```python
from build123d import *
from build123d.topology import SkipClean

# Parameters (mm, degrees)
SKETCH_1_R          = 22
SKETCH_1_R_2        = 11.15
SKETCH_1_R_3        = 2.7
EXTRUDE_1_DEPTH     = 10
EXTRUDE_START       = -10
EXTRUDE_2_DEPTH     = 10
CUT_EXTRUDE_START   = -10
CUT_EXTRUDE_1_DEPTH = 10
SKETCH_4_W          = 20
SKETCH_4_H          = 20
EXTRUDE_3_DEPTH     = 15
CHAMFER_2_SIZE      = 10
CHAMFER_4_SIZE      = 1
SKETCH_6_R          = 1.7
CUT_EXTRUDE_3_DEPTH = 92.290744328
CHAMFER_6_SIZE      = 1


with BuildPart() as part:
    # ｽｹｯﾁ1 → ﾎﾞｽ - 押し出し1 (new body)
    with BuildSketch(Plane.XY):
        Circle(SKETCH_1_R)
        Circle(SKETCH_1_R_2, mode=Mode.SUBTRACT)
        with Locations((-8.75, -15.155444566)):
            Circle(SKETCH_1_R_3, mode=Mode.SUBTRACT)
        with Locations((17.5, 0)):
            Circle(SKETCH_1_R_3, mode=Mode.SUBTRACT)
        with Locations((-8.75, 15.155444566)):
            Circle(SKETCH_1_R_3, mode=Mode.SUBTRACT)
    extrude(amount=EXTRUDE_1_DEPTH)

    # ｽｹｯﾁ2 → ﾎﾞｽ - 押し出し2 (add)
    with BuildSketch(Plane.XY.offset(10).offset(EXTRUDE_START)):
        with BuildLine():
            ThreePointArc((0, -22), (-22, 0), (0, 22))
            Line((0, 22), (-85, 22))
            Line((-85, 22), (-85, -22))
            Line((-85, -22), (0, -22))
        make_face()
    extrude(amount=EXTRUDE_2_DEPTH)

    # ｽｹｯﾁ3 → ｶｯﾄ - 押し出し1 (cut)
    with BuildSketch(Plane.XY.offset(10).offset(CUT_EXTRUDE_START)):
        with BuildLine():
            Line((-85, 22), (-85, 10))
            Line((-85, 10), (-19.595917942, 10))
            ThreePointArc((-19.595917942, 10), (-11.489125293, 18.761663039), (0, 22))
            Line((0, 22), (-85, 22))
        make_face()
        with BuildLine():
            Line((-19.595917942, -10), (-85, -10))
            Line((-85, -10), (-85, -22))
            Line((-85, -22), (0, -22))
            ThreePointArc((0, -22), (-11.489125293, -18.761663039), (-19.595917942, -10))
        make_face()
    extrude(amount=CUT_EXTRUDE_1_DEPTH, mode=Mode.SUBTRACT)

    # ｽｹｯﾁ4 → ﾎﾞｽ - 押し出し3 (add)
    with BuildSketch(Plane(origin=(0, 0, 0), x_dir=(-1, 0, 0), z_dir=(0, 0, -1))):
        with Locations((75, 0)):
            Rectangle(SKETCH_4_W, SKETCH_4_H)
    extrude(amount=EXTRUDE_3_DEPTH)

    # 面取り2
    chamfer_2_edges = [part.edges().sort_by_distance(p)[0] for p in [
        (-65, 0, 0),
    ]]
    chamfer(chamfer_2_edges, length=CHAMFER_2_SIZE)

    # 面取り4
    chamfer_4_edges = [part.edges().sort_by_distance(p)[0] for p in [
        (22, 0, 10),
        (-52.297958971, 10, 10),
        (-52.297958971, -10, 10),
    ]]
    chamfer(chamfer_4_edges, length=CHAMFER_4_SIZE)

    # ｽｹｯﾁ6 → ｶｯﾄ - 押し出し3 (cut, through all)
    with SkipClean():  # the faces are left unmerged after this step: merging them gives an invalid solid
        with BuildSketch(Plane(origin=(0, 0, -15), x_dir=(-1, 0, 0), z_dir=(0, 0, -1))):
            with Locations((80, 5)):
                Circle(SKETCH_6_R)
            with Locations(Location((70, 5, 0), (0, 0, 180))):
                Circle(SKETCH_6_R)
            with Locations((70, -5)):
                Circle(SKETCH_6_R)
            with Locations(Location((80, -5, 0), (0, 0, 180))):
                Circle(SKETCH_6_R)
        extrude(amount=-CUT_EXTRUDE_3_DEPTH, mode=Mode.SUBTRACT)

    # 面取り6
    chamfer_6_edges = [part.edges().sort_by_distance(p)[0] for p in [
        (-85, 0, 10),
    ]]
    chamfer(chamfer_6_edges, length=CHAMFER_6_SIZE)


solid = part.part
```
Geometry: final body of the model. Coordinates: model frame, mm. A direction names the side the tool comes from. Coordinates: 2 decimals unless noted, no trailing zeros. Order: outer loops, then holes, each group sorted by start corner. A loop starts at its lowest first (then second) coordinate and runs counter-clockwise, first axis right, second up. Notation, with made-up numbers: (14, 50.5) -> (32, 50.5) arc R18 ccw to (32, 62.5) -> close; hole circle Ø6 at (-27, -33.75). An arc over 180 degrees is marked (long way). Write item = value, one per line.
(1) Pin query (flat end, axial travel): pin 1 Ø6 at (x, z) = (-38.5, 2) entering from -Y; pin 2 Ø8.5 at (x, y) = (17.5, 0) entering from +Z; pin 3 Ø22 at (x, y) = (-18.5, 4) entering from -Z; pin 4 Ø5.5 at (y, z) = (3.5, -12.5) entering from +X. Return the tip coordinate at first contact, or that it passes through.
Solved:
pin_1 = -10
pin_2 = 10
pin_3 = 0
pin_4 = -64.75
(2) Line query: line 1 (Y direction, x = -70, z = -8); line 2 (X direction, y = -4, z = -2); line 3 (X direction, y = 1.5, z = 8) (3 decimals). Output: solid intervals per line, ascending.
Solved:
line_1 = -10 to -6.7, -3.3 to 3.3, 6.7 to 10
line_2 = -85 to -81.37, -78.63 to -71.37, -68.63 to -57
line_3 = -85 to -11.049, 11.049 to 15.255, 19.745 to 21.949
(3) Cut plane C-C on z = -13. Return loops of the section in (x, y).
Solved:
outline = (-85, -10) -> (-65, -10) -> (-65, 10) -> (-85, 10) -> close; hole circle Ø3.4 at (-80, -5); hole circle Ø3.4 at (-80, 5); hole circle Ø3.4 at (-70, -5); hole circle Ø3.4 at (-70, 5)
(4) Pull-direction query (Y, two-part tool) for faces 1 (the flat face through (-65, 0, -12)), 2 (the flat face through (-59, -10, 0)), 3 (the cylindrical face through (10.635, 3.349, 4.93)); classes: pulls with the +Y half, pulls with the -Y half, needs draft (parallel to the pull), parting line crosses it, or undercut.
Solved:
face_1 = needs draft
face_2 = pulls with the -Y half
face_3 = undercut
(5) Cut plane A-A on y = 0. Return loops of the section in (x, z), plus the area to 3 significant figures.
Solved:
outline = (-85, -15) -> (-65, -15) -> (-65, -10) -> (-55, 0) -> (-11.15, 0) -> (-11.15, 10) -> (-84, 10) -> (-85, 9) -> close; (11.15, 0) -> (14.8, 0) -> (14.8, 10) -> (11.15, 10) -> close; (20.2, 0) -> (22, 0) -> (22, 9) -> (21, 10) -> (20.2, 10) -> close
area = 1,140 mm²
(6) Access query for faces 4 (the flat face through (-59, 10, 0)), 5 (the cylindrical face through (-68.3, -4.93, -2.68)), 6 (the flat face through (-17, 0, 0)). Directions: +Z, -Z, +X, -X, +Y, -Y. A direction counts if a zero-diameter tool reaches every point of the face in a straight line with its end or side. Return the directions, or none.
Solved:
face_4 = +Z, -Z, -X, +Y
face_5 = +Z, -Z
face_6 = -Z, +X, +Y, -Y
(7) Cut plane D-D on z = -4. Return loops of the section in (x, y), plus the area to 3 significant figures.
Solved:
outline = (-85, -10) -> (-59, -10) -> (-59, 10) -> (-85, 10) -> close; hole circle Ø3.4 at (-80, -5); hole circle Ø3.4 at (-80, 5); hole circle Ø3.4 at (-70, -5); hole circle Ø3.4 at (-70, 5)
area = 484 mm²
(8) Cut plane B-B on x = -70. Return loops of the section in (y, z), plus the area to 3 significant figures.
Solved:
outline = (-10, -15) -> (-6.7, -15) -> (-6.7, 10) -> (-9, 10) -> (-10, 9) -> close; (-3.3, -15) -> (3.3, -15) -> (3.3, 10) -> (-3.3, 10) -> close; (6.7, -15) -> (10, -15) -> (10, 9) -> (9, 10) -> (6.7, 10) -> close
area = 329 mm²
